Geometry check sheet. Reference: drawing and pictorial views, mm from the part's lowest x, y, z. A direction names the side the tool comes from. Round coordinates to 2 decimals unless told otherwise and drop trailing zeros. Loops run counter-clockwise (first coordinate to the right, second up) from the corner with the lowest first, then second, coordinate; pieces in that order, holes last. Notation, with made-up numbers: (85, -39.5) -> (91, -39.5) arc R6 ccw to (91, -34.5) -> close; hole circle Ø5 at (-23, 32). An arc over 180 degrees is marked (long way). Write item = value, one per line.
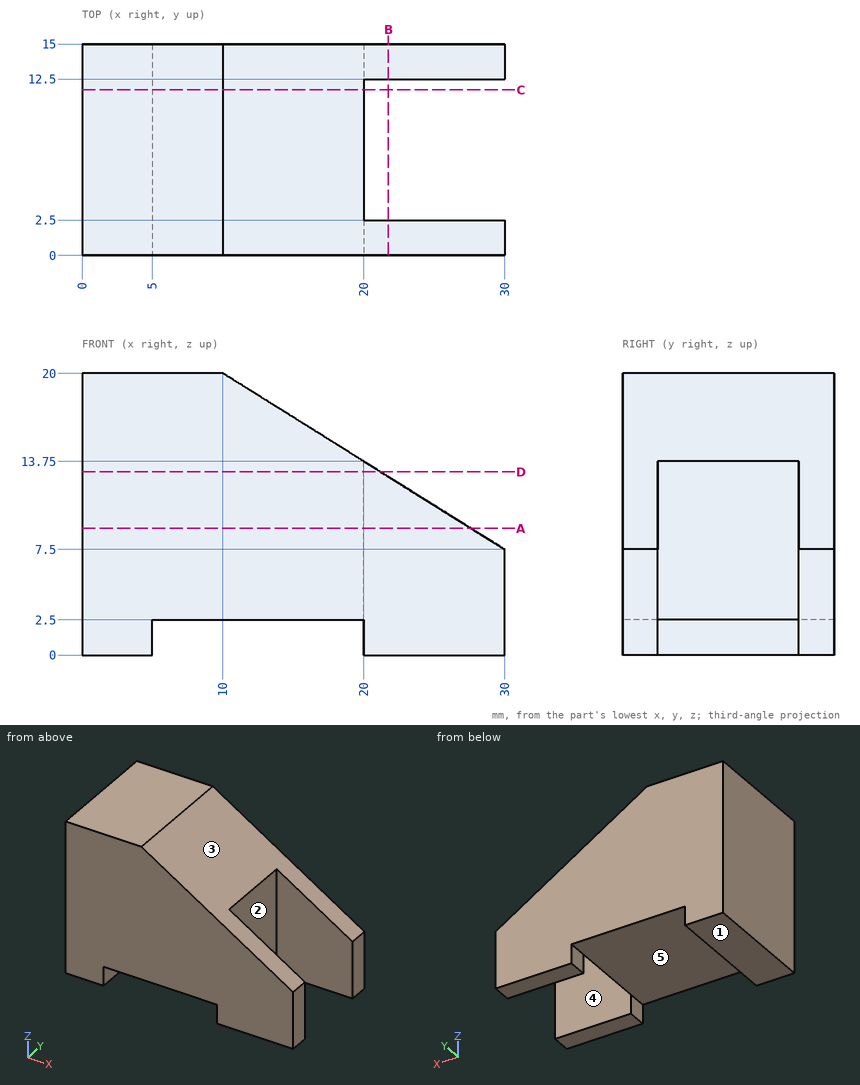
(1) Sectioned sample at C-C, the plane y = 11.75. Record the cut outline in (x, z), and give its area (3 significant figures).
Filled sheet:
outline = (0, 0) -> (5, 0) -> (5, 2.5) -> (20, 2.5) -> (20, 13.75) -> (10, 20) -> (0, 20) -> close
area = 331 mm2
(2) Go/stop test with flat-tipped pins: pin 1 Ø8 at (x, y) = (17.5, 4) entering from +Z; pin 2 Ø4 at (x, y) = (20.5, 1.5) entering from +Z. Record where each tip stops, or that it passes through.
Filled sheet:
pin_1 = 17.81
pin_2 = 14.69
(3) Sectioned sample at D-D, the plane z = 13. Record the cut outline in (x, y), and give its area (3 significant figures).
Filled sheet:
outline = (0, 0) -> (21.2, 0) -> (21.2, 2.5) -> (20, 2.5) -> (20, 12.5) -> (21.2, 12.5) -> (21.2, 15) -> (0, 15) -> close
area = 306 mm2
(4) Material ranges on probe 1 along Y at (x, z) = (21, 1.25); probe 2 along X at (y, z) = (10, 6.75); probe 3 along X at (y, z) = (13, 1.75), recorded low to high. Write a range as from..to.
Filled sheet:
probe_1 = 0..2.5, 12.5..15
probe_2 = 0..20
probe_3 = 0..5, 20..30
(5) Set-up check for the marked faces 1 and 2: record each of +Z, -Z, +X, -X, +Y, -Y from which the full face is reachable in a straight line by a thin tool's end or side.
Filled sheet:
face_1 = -Z, +X, -X, +Y, -Y
face_2 = +Z, -Z, +X
(6) Sectioned sample at B-B, the plane x = 21.75. Record the cut outline in (y, z), and give its area (3 significant figures).
Filled sheet:
outline = (0, 0) -> (2.5, 0) -> (2.5, 12.66) -> (0, 12.66) -> close; (12.5, 0) -> (15, 0) -> (15, 12.66) -> (12.5, 12.66) -> close
area = 63.3 mm2
(7) Draft check along X on the marked faces 3, 4 and 5. Enter one of: released by +X, released by -X, zero draft, split by the parting line, or undercut.
Filled sheet:
face_3 = released by +X
face_4 = zero draft
face_5 = undercut
(8) Sectioned sample at A-A, the plane z = 9. Record the cut outline in (x, y), and give its area (3 significant figures).
Filled sheet:
outline = (0, 0) -> (27.6, 0) -> (27.6, 2.5) -> (20, 2.5) -> (20, 12.5) -> (27.6, 12.5) -> (27.6, 15) -> (0, 15) -> close
area = 338 mm2
